from build123d import *

# Parameters (mm, degrees)
SKETCH1_R           = 14.25
SKETCH1_R_2         = 1.7
BOSS_EXTRUDE1_DEPTH = 3.175
SKETCH5_R           = 1.25
CUT_EXTRUDE4_DEPTH  = 4.175
CUT_EXTRUDE5_DEPTH  = 10
FILLET1_R           = 5
FILLET2_R           = 5


with BuildPart() as part:
    # Sketch1 → Boss-Extrude1 (new body)
    with BuildSketch(Plane.XY):
        with BuildLine():
            Line((-72.715301765, 90.837326721), (-152.817002247, 126.544575004))
            ThreePointArc((-152.817002247, 126.544575004), (-157.784388135, 127.370762315), (-162.524605276, 125.671394934))
            Line((-162.524605276, 125.671394934), (-222.299360222, 152.317421212))
            ThreePointArc((-222.299360222, 152.317421212), (-249.039738928, 142.066706765), (-238.78902448, 115.326328059))
            Line((-238.78902448, 115.326328059), (-179.014269534, 88.680301782))
            ThreePointArc((-179.014269534, 88.680301782), (-177.109561802, 84.018800254), (-173.174612442, 80.876558766))
            Line((-173.174612442, 80.876558766), (-93.072911961, 45.169310483))
            ThreePointArc((-93.072911961, 45.169310483), (-85.421957972, 44.965480094), (-79.867786674, 50.231391692))
            Line((-79.867786674, 50.231391692), (-67.653220557, 77.632201435))
            ThreePointArc((-67.653220557, 77.632201435), (-67.449390168, 85.283155423), (-72.715301765, 90.837326721))
        make_face()
        with Locations((-230.544192351, 133.821874636)):
            Circle(SKETCH1_R, mode=Mode.SUBTRACT)
        with Locations((-95.571468701, 49.02024728)):
            Circle(SKETCH1_R_2, mode=Mode.SUBTRACT)
        with Locations((-132.105881692, 65.306335437)):
            Circle(SKETCH1_R_2, mode=Mode.SUBTRACT)
        with Locations((-168.640294682, 81.592423593)):
            Circle(SKETCH1_R_2, mode=Mode.SUBTRACT)
        with Locations((-150.318445506, 122.693638207)):
            Circle(SKETCH1_R_2, mode=Mode.SUBTRACT)
        with Locations((-113.784032516, 106.407550051)):
            Circle(SKETCH1_R_2, mode=Mode.SUBTRACT)
        with Locations((-77.249619525, 90.121461895)):
            Circle(SKETCH1_R_2, mode=Mode.SUBTRACT)
        with Locations((-81.295075004, 54.152214057)):
            Circle(SKETCH1_R_2, mode=Mode.SUBTRACT)
        with Locations((-71.52342211, 76.072861852)):
            Circle(SKETCH1_R_2, mode=Mode.SUBTRACT)
        with Locations((-168.932649456, 106.357056211)):
            Circle(SKETCH1_R_2, mode=Mode.SUBTRACT)
    extrude(amount=BOSS_EXTRUDE1_DEPTH)

    # Sketch5 → Cut-Extrude4 (cut, through all)
    with BuildSketch(Plane.XY.offset(3.175)):
        with Locations((-196.466353254, 99.744559857)):
            Circle(SKETCH5_R)
        with Locations((-224.780523322, 112.366278179)):
            Circle(SKETCH5_R)
        with Locations((-210.733772287, 143.877209383)):
            Circle(SKETCH5_R)
        with Locations((-182.419602219, 131.255491062)):
            Circle(SKETCH5_R)
        with Locations((-242.947351213, 145.810375386)):
            Circle(SKETCH5_R)
        with Locations((-247.751623016, 135.033002179)):
            Circle(SKETCH5_R)
    extrude(amount=-CUT_EXTRUDE4_DEPTH, mode=Mode.SUBTRACT)

    # Sketch6 → Cut-Extrude5 (cut)
    with BuildSketch(Plane.XY.offset(3.175)):
        Polygon((-158.059591703, 123.407293834), (-70.184261161, 84.234764078), (-86.470349317, 47.700351088), (-174.345679859, 86.872880843), align=None)
    extrude(amount=-CUT_EXTRUDE5_DEPTH, mode=Mode.SUBTRACT)

    # Fillet1
    fillet1_edges = [part.edges().sort_by_distance(p)[0] for p in [
        (-174.345679859, 86.872880843, 1.5875),
        (-158.059591703, 123.407293834, 1.5875),
    ]]
    fillet(fillet1_edges, radius=FILLET1_R)

    # Fillet2
    fillet2_edges = [part.edges().sort_by_distance(p)[0] for p in [
        (-70.184261161, 84.234764078, 1.5875),
        (-86.470349317, 47.700351088, 1.5875),
    ]]
    fillet(fillet2_edges, radius=FILLET2_R)


solid = part.part
The listing builds one solid part. Answer for the finished solid, in the listing's coordinates (mm). A direction names the side the tool comes from. Round coordinates to 2 decimals unless told otherwise and drop trailing zeros. Write each loop counter-clockwise with the first axis right and the second up, starting at its lowest first coordinate (ties: lowest second). Pieces come first, ordered by that corner, then holes. Notation, with made-up numbers: M 63.5,61 L 71.5,61 A12 cw 71.5,77 Z; hole C 32,12.5 d2. An arc over 180 degrees is marked long. Write each question's results on one line, items separated by ' | '. Start each with the question number.
Item 1: A cutting plane is placed at D-D on x = -177. Write down the section's boundary in (y, z) (3 decimals).
Item 2: A cutting plane is placed at B-B on z = 2.05. State how many separate pieces and enclosed holes the cut face has, and give its area (3 significant figures).
Item 3: A cutting plane is placed at C-C on y = 71. Write down the section's boundary in (x, z) (3 decimals), and give its area (3 significant figures).
Item 4: For a pull along X with two mould halves and no side action, classify faces 3 (the face through (-85.52, 44.93, 1.57)), 4 (the face through (-177.152, 84.076, 1.565)), 5 (the face through (-82.644, 53.118, 1.565)) as pulls with the +X half, pulls with the -X half, needs draft (parallel to the pull), parting line crosses it, or undercut.
Item 5: A cutting plane is placed at A-A on x = -138.5. Write down the section's boundary in (y, z) (3 decimals).
Item 6: Straight lines are drawn through the part: L1, parallel to X at y = 80.5, z = 0.3; L2, parallel to X at y = 59.5, z = 1.15; L3, parallel to X at y = 72, z = 2.9. For each, find the intervals that lie inside material, in ascending order. Write a range as [from, to].
Item 7: For faces 1 (the face through (-78.24, 66.16, 1.61)), 2 (the face through (-180, 108, 0)), determine the directions among +Z, -Z, +X, -X, +Y, -Y from which every point of the face is accessible in a straight line to the end or side of a thin tool.
Check sheet entries:
1) outline: M 83.875,0 L 132.124,0 L 132.124,3.175 L 83.875,3.175 Z
2) separate pieces: 1 | enclosed holes: 17 | area: 3,960 mm²
3) outline: M -151.019,0 L -138.738,0 L -138.738,3.175 L -151.019,3.175 Z; M -76.084,0 L -70.61,0 L -70.61,3.175 L -76.084,3.175 Z | area: 56.4 mm²
4) face 3: parting line crosses it | face 4: pulls with the -X half | face 5: undercut
5) outline: M 65.42,0 L 70.894,0 L 70.894,3.175 L 65.42,3.175 Z; M 114.688,0 L 120.162,0 L 120.162,3.175 L 114.688,3.175 Z
6) L1: [-172.33, -169.94], [-167.34, -160.05], [-71.93, -66.86] | L2: [-125.22, -112.94], [-81.21, -75.74] | L3: [-153.26, -140.98], [-75.64, -70.16]
7) face 1: +Z, -Z | face 2: -Z, +X, -X, +Y, -Y
